```python
from build123d import *

# Parameters (mm, degrees)
SKETCH1_R           = 5
BOSS_EXTRUDE1_DEPTH = 25
SKETCH2_R           = 2.1
CUT_EXTRUDE1_DEPTH  = 10
SKETCH3_W           = 2
SKETCH3_H           = 6.2
CUT_EXTRUDE2_DEPTH  = 10


with BuildPart() as part:
    # Sketch1 → Boss-Extrude1 (new body)
    with BuildSketch(Plane.XY):
        Circle(SKETCH1_R)
    extrude(amount=BOSS_EXTRUDE1_DEPTH)

    # Sketch2 → Cut-Extrude1 (cut)
    with BuildSketch(Plane.XY.offset(25)):
        Circle(SKETCH2_R)
    extrude(amount=-CUT_EXTRUDE1_DEPTH, mode=Mode.SUBTRACT)

    # Sketch3 → Cut-Extrude2 (cut)
    with BuildSketch(Plane.XY.offset(25)):
        Rectangle(SKETCH3_W, SKETCH3_H)
    extrude(amount=-CUT_EXTRUDE2_DEPTH, mode=Mode.SUBTRACT)


solid = part.part
```
Geometry check sheet. Reference: the model listing, model coordinates, mm. A direction names the side the tool comes from. Round coordinates to 2 decimals unless told otherwise and drop trailing zeros. Order: outer loops, then holes, each group sorted by start corner. A loop starts at its lowest first (then second) coordinate and runs counter-clockwise, first axis right, second up. Notation, with made-up numbers: (34, 48.25) - (69, 48.25) arc R20 ccw to (69, 55.25) - close; hole circle Ø5 at (-6, -31). An arc over 180 degrees is marked (long way). Use a Markdown table: item, result. Add a question column.
(1) Release check for a two-part mould opening along X. For faces 1 (the flat face through (0, 0, 0)), 2 (the flat face through (0, -3.1, 20)), 3 (the cylindrical face through (-1.08, -4.88, 12.32)) record: pulls with the +X half, pulls with the -X half, needs draft (parallel to the pull), parting line crosses it, or undercut.
(2) Material ranges on line 1 along Y through (x, z) = (-0.75, 21.5); line 2 along X through (y, z) = (2.75, 16.75); line 3 along X through (y, z) = (1.5, 15.5), recorded low to high. Write a range as [from, to].
(3) Tool access check on faces 4 (the flat face through (0, 3.1, 20)), 5 (the flat face through (2.2, -1, 25)). Record the directions out of +Z, -Z, +X, -X, +Y, -Y that give a thin tool (end or side, any length) a straight path to the whole face; none if there is none.
(4) Sectioned sample at C-C, the plane x = 0. Enter the section's corners in (y, z), and give its area (3 significant figures).
(5) Sectioned sample at D-D, the plane z = 7. Enter the section's corners in (x, y).
(6) Sectioned sample at B-B, the plane y = 0. Enter the section's corners in (x, z), and give its area (3 significant figures).
(7) Sectioned sample at A-A, the plane z = 17. Enter the section's corners in (x, y).
(8) Depth check by flat-ended pin: pin 1 (2 mm diameter, centred on x = -3, z = 21.5, fed in from -Y); pin 2 (0.6 mm diameter, centred on y = 2.5, z = 18.5, fed in from -X); pin 3 (2 mm diameter, centred on x = 1, y = 0, fed in from +Z). Enter the tip coordinate at first touch or a pass-through.
Answers below:
| question | item | result |
|---|---|---|
| 1 | face 1 | needs draft |
| 1 | face 2 | undercut |
| 1 | face 3 | parting line crosses it |
| 2 | line 1 | [-4.94, -3.1], [3.1, 4.94] |
| 2 | line 2 | [-4.18, -1], [1, 4.18] |
| 2 | line 3 | [-4.77, -1.47], [1.47, 4.77] |
| 3 | face 4 | +Z |
| 3 | face 5 | +Z, +X, -X, +Y, -Y |
| 4 | outline | (-5, 0) - (5, 0) - (5, 25) - (3.1, 25) - (3.1, 15) - (-3.1, 15) - (-3.1, 25) - (-5, 25) - close |
| 4 | area | 188 mm² |
| 5 | outline | circle Ø10 at (0, 0) |
| 6 | outline | (-5, 0) - (5, 0) - (5, 25) - (2.1, 25) - (2.1, 15) - (-2.1, 15) - (-2.1, 25) - (-5, 25) - close |
| 6 | area | 208 mm² |
| 7 | outline | circle Ø10 at (0, 0); hole (-1, -3.1) - (1, -3.1) - (1, -1.85) arc R2.1 ccw to (1, 1.85) - (1, 3.1) - (-1, 3.1) - (-1, 1.85) arc R2.1 ccw to (-1, -1.85) - close |
| 8 | pin 1 | y = -4.58 |
| 8 | pin 2 | x = -4.49 |
| 8 | pin 3 | z = 15 |
